Here's how the part is built. I have some questions about the finished solid (model axes, mm). Face numbers are marked on the shaded views. A direction names the side the tool comes from. Coordinates: 2 decimals unless noted, no trailing zeros. Order: outer loops, then holes, each group sorted by start corner. A loop starts at its lowest first (then second) coordinate and runs counter-clockwise, first axis right, second up. Notation, with made-up numbers: (75, 43) - (127, 43) arc R32 ccw to (127, 78) - close; hole circle Ø11 at (68.5, 28). An arc over 180 degrees is marked (long way). Answer as CSV lines item,"result". Start each with the question number.
Item 1: I'm going to push flat-ended pins straight in: pin 1 (5 mm diameter, centred on y = 5.5, z = 7, fed in from -X); pin 2 (5 mm diameter, centred on y = 9.5, z = 9, fed in from +X); pin 3 (1.1 mm diameter, centred on x = -15.5, z = 19, fed in from -Y); pin 4 (12 mm diameter, centred on x = 13, z = 11, fed in from +Y). Where does each tip first touch, or does it pass through?
Item 2: I need wall thicknesses on line 1 (X direction, y = 7.5, z = -15.5); line 2 (X direction, y = 1.5, z = 15); line 3 (X direction, y = 7, z = 10). Which ranges of each line are inside material? Lowest first, please.
Item 3: Imagine slicing it at B-B on x = 15.5. List the corners of the cut face in (y, z) for me.
Item 4: On a 3-axis mill with a long thin cutter (end or side, diameter ignored), from which of +Z, -Z, +X, -X, +Y, -Y can I reach the whole of each face in a straight line? I mean the marked faces 1 and 2. Say none if no direction works.
Item 5: Imagine slicing it at C-C on z = 15.5. List the corners of the cut face in (x, y) for me.
Item 6: Imagine slicing it at A-A on y = 5.5. List the corners of the cut face in (x, z) for me.
Item 7: We'd pull the mould along X, two halves only. Please class the marked faces 3, 4 and 5: pulls with the +X half, pulls with the -X half, needs draft (parallel to the pull), parting line crosses it, or undercut.
Item 8: Imagine slicing it at D-D on x = -11. List the corners of the cut face in (y, z) for me, and give its area (3 significant figures).
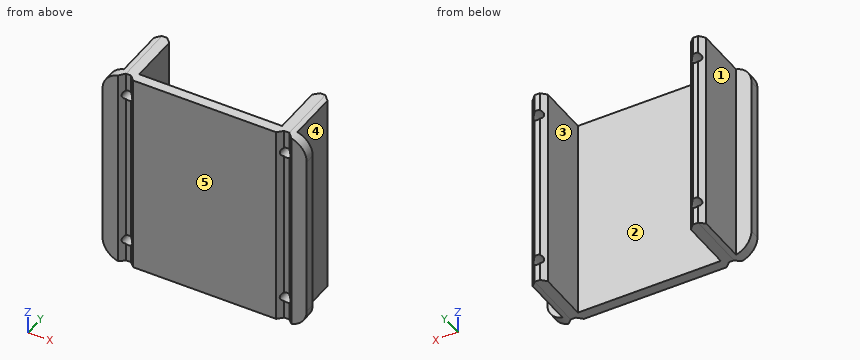
from build123d import *

# Parameters (mm, degrees)
SKETCH1_W           = 40
SKETCH1_H           = 40
BOSS_EXTRUDE1_DEPTH = 2
CUT_EXTRUDE1_DEPTH  = 45.766058571
BOSS_EXTRUDE2_START = -40
BOSS_EXTRUDE2_DEPTH = 40
FILLET1_R           = 4
SKETCH6_R           = 1.05
CUT_EXTRUDE4_DEPTH  = 32.128764833


with BuildPart() as part:
    # Sketch1 → Boss-Extrude1 (new body)
    with BuildSketch(Plane(origin=(0, 0, 0), x_dir=(1, 0, 0), z_dir=(0, 1, 0))):
        Rectangle(SKETCH1_W, SKETCH1_H)
    extrude(amount=BOSS_EXTRUDE1_DEPTH)

    # Sketch2 → Cut-Extrude1 (cut, through all)
    with BuildSketch(Plane.XY.offset(20)):
        Polygon((14, 0), (15, 1), (16, 1), (17, 0), align=None)
    cut_extrude1 = extrude(amount=-CUT_EXTRUDE1_DEPTH, mode=Mode.SUBTRACT)

    # Sketch3 → Boss-Extrude2 (add)
    with BuildSketch(Plane.XY.offset(20).offset(BOSS_EXTRUDE2_START)):
        Polygon((17, 12), (16, 13), (15, 13), (14, 12), (14, 2), (17, 2), align=None)
    boss_extrude2 = extrude(amount=BOSS_EXTRUDE2_DEPTH)

    # Mirror2: Cut-Extrude1, Boss-Extrude2 across plane
    add(cut_extrude1.mirror(Plane(origin=(0, 0, 0), x_dir=(0, 0, 1), z_dir=(1, 0, 0))), mode=Mode.SUBTRACT)
    add(boss_extrude2.mirror(Plane(origin=(0, 0, 0), x_dir=(0, 0, 1), z_dir=(1, 0, 0))))

    # Fillet1
    fillet1_edges = [part.edges().sort_by_distance(p)[0] for p in [
        (-20, 1, 20),
        (20, 1, 20),
        (20, 1, -20),
        (-20, 1, -20),
    ]]
    fillet(fillet1_edges, radius=FILLET1_R)

    # Sketch6 → Cut-Extrude4 (cut, through all)
    with BuildSketch(Plane(origin=(0, 0, 0), x_dir=(1, 0, 0), z_dir=(0, 1, 0))):
        with Locations(Location((-15.5, 15.5, 0), (0, 0, 61.563109851))):
            Circle(SKETCH6_R)
        with Locations(Location((15.5, 15.5, 0), (0, 0, 61.563109851))):
            Circle(SKETCH6_R)
        with Locations(Location((-15.5, -15.5, 0), (0, 0, 61.563109851))):
            Circle(SKETCH6_R)
        with Locations(Location((15.5, -15.5, 0), (0, 0, 61.563109851))):
            Circle(SKETCH6_R)
    extrude(amount=CUT_EXTRUDE4_DEPTH, mode=Mode.SUBTRACT)


solid = part.part
Responses:
1,pin 1,"stops at x = -17"
1,pin 2,"stops at x = 17"
1,pin 3,"stops at y = 0.95"
1,pin 4,"stops at y = 13"
2,line 1,"x = -17 to -16.55, -14.45 to -14, 14 to 14.45, 16.55 to 17"
2,line 2,"x = -20 to -16.42, -14.58 to 14.58, 16.42 to 20"
2,line 3,"x = -17 to -14, 14 to 17"
3,outline,"(1, -20) - (13, -20) - (13, -16.55) - (1, -16.55) - close; (1, -14.45) - (13, -14.45) - (13, 14.45) - (1, 14.45) - close; (1, 16.55) - (13, 16.55) - (13, 20) - (1, 20) - close"
4,face 1,"+Z, -Z, -X, +Y"
4,face 2,"+Z, -Z, +Y"
5,outline,"(-20, 0) - (-17, 0) - (-16.55, 0.45) - (-16.55, 12.45) - (-17, 12) - (-17, 2) - (-20, 2) - close; (-14.45, 0.45) - (-14, 0) - (14, 0) - (14.45, 0.45) - (14.45, 12.45) - (14, 12) - (14, 2) - (-14, 2) - (-14, 12) - (-14.45, 12.45) - close; (16.55, 0.45) - (17, 0) - (20, 0) - (20, 2) - (17, 2) - (17, 12) - (16.55, 12.45) - close"
6,outline,"(-17, -19.87) arc R4 ccw to (-16, -20) - (-14, -20) - (-14, 20) - (-16, 20) arc R4 ccw to (-17, 19.87) - close; (14, -20) - (16, -20) arc R4 ccw to (17, -19.87) - (17, 19.87) arc R4 ccw to (16, 20) - (14, 20) - close; hole circle Ø2.1 at (-15.5, -15.5); hole circle Ø2.1 at (-15.5, 15.5); hole circle Ø2.1 at (15.5, -15.5); hole circle Ø2.1 at (15.5, 15.5)"
7,face 3,"undercut"
7,face 4,"pulls with the +X half"
7,face 5,"needs draft"
8,outline,"(0, -20) - (2, -20) - (2, 20) - (0, 20) - close"
8,area,"80.0 mm^2"
